CAD build for the part. Positions are in the model's coordinates, mm. A direction names the side the tool comes from. Coordinates: 2 decimals unless noted, no trailing zeros. Write each loop counter-clockwise with the first axis right and the second up, starting at its lowest first coordinate (ties: lowest second). Pieces come first, ordered by that corner, then holes. Notation, with made-up numbers: (-34.75, 42.25) - (-20.75, 42.25) arc R27 cw to (-20.75, 76.25) - close; hole circle Ø2 at (47, 70). An arc over 180 degrees is marked (long way). Answer in a Markdown table with one row per item. Add a question column.
Q1. Band-saw the part on C-C (z = -10.75). List the corners of the cut face in (x, y) (3 decimals), and give its area (3 significant figures).
Q2. Two-plate mould, pull along X, no slides. Class faces 1 (the flat face through (-3, 27.813, -10)), 2 (the cylindrical face through (-4.48, 29.42, -2.52)), 3 (the flat face through (0, 34, -10)): +X half, -X half, draft (parallel to the pull), parting line (faces both ways), or undercut.
Q3. 3-axis set-ups, long thin cutter, end or side, ignore diameter. For faces 4 (the flat face through (0, 14, -10)), 5 (the flat face through (-3, 30.988, -10)), 6 (the flat face through (40.005, 14, -10)): which of +Z, -Z, +X, -X, +Y, -Y reach the whole face in a straight line?
Q4. Band-saw the part on A-A (z = -5.25). List the corners of the cut face in (x, y) (3 decimals).
Q5. Pin check, flat tips, straight feed: pin 1 (10 mm diameter, centred on y = 6, z = -6, fed in from +X) (3 decimals); pin 2 (5 mm diameter, centred on x = 24.5, y = 21, fed in from +Z); pin 3 (5 mm diameter, centred on x = 28, z = -12, fed in from +Y); pin 4 (4 mm diameter, centred on y = 24.5, z = -15, fed in from -X). Stop position of each tip, or through.
Q6. Band-saw the part on D-D (x = 11). List the corners of the cut face in (y, z), and give its area (3 significant figures).
Q7. Drill centre lines: line 1 along Y through (x, z) = (25, -4.25); line 2 along X through (y, z) = (16, -18.5) (3 decimals); line 3 along Y through (x, z) = (43, -18.5). Where is each one in solid material? Low to high. Write a range as from..to.
Q8. Band-saw the part on B-B (y = 19). List the corners of the cut face in (x, z) (3 decimals).
```python
from build123d import *

# Parameters (mm, degrees)
SKETCH1_W           = 40.005
SKETCH1_H           = 19.939
BOSS_EXTRUDE1_DEPTH = 37.338
SKETCH2_W           = 19.939
SKETCH2_H           = 3.175
BOSS_EXTRUDE2_DEPTH = 7.62
SKETCH3_R           = 2.2225
CUT_EXTRUDE1_DEPTH  = 61.215948801
SKETCH4_R           = 2.921
BOSS_EXTRUDE3_DEPTH = 8.636


with BuildPart() as part:
    # Sketch1 → Boss-Extrude1 (new body)
    with BuildSketch(Plane(origin=(0, 0, 0), x_dir=(1, 0, 0), z_dir=(0, 1, 0))):
        with Locations((20.0025, 9.9695)):
            Rectangle(SKETCH1_W, SKETCH1_H)
    extrude(amount=BOSS_EXTRUDE1_DEPTH)

    # Sketch2 → Boss-Extrude2 (add)
    with BuildSketch(Plane(origin=(40.005, 0, 0), x_dir=(0, 0, -1), z_dir=(1, 0, 0))):
        with Locations((9.9695, 29.4005)):
            Rectangle(SKETCH2_W, SKETCH2_H)
    boss_extrude2 = extrude(amount=BOSS_EXTRUDE2_DEPTH)

    # Sketch3 → Cut-Extrude1 (cut, through all)
    with BuildSketch(Plane(origin=(0, 30.988, 0), x_dir=(1, 0, 0), z_dir=(0, 1, 0))):
        with Locations(Location((45.339, 15.367, 0), (0, 0, 270))):
            Circle(SKETCH3_R)
        with Locations(Location((45.339, 4.572, 0), (0, 0, 270))):
            Circle(SKETCH3_R)
    cut_extrude1 = extrude(amount=-CUT_EXTRUDE1_DEPTH, mode=Mode.SUBTRACT)

    # Mirror1: Boss-Extrude2, Cut-Extrude1 across plane
    add(boss_extrude2.mirror(Plane(origin=(20.0025, 0, 0), x_dir=(0, 0, 1), z_dir=(1, 0, 0))))
    add(cut_extrude1.mirror(Plane(origin=(20.0025, 0, 0), x_dir=(0, 0, 1), z_dir=(1, 0, 0))), mode=Mode.SUBTRACT)

    # Sketch4 → Boss-Extrude3 (add)
    with BuildSketch(Plane(origin=(0, 37.338, 0), x_dir=(1, 0, 0), z_dir=(0, 1, 0))):
        with Locations(Location((9.779, 9.9695, 0), (0, 0, 90))):
            Circle(SKETCH4_R)
    extrude(amount=BOSS_EXTRUDE3_DEPTH)


solid = part.part
```
Checked values:
| question | item | result |
|---|---|---|
| 1 | outline | (-7.62, 27.813) - (0, 27.813) - (0, 0) - (40.005, 0) - (40.005, 27.813) - (47.625, 27.813) - (47.625, 30.988) - (40.005, 30.988) - (40.005, 37.338) - (12.594, 37.338) - (12.594, 45.974) - (6.964, 45.974) - (6.964, 37.338) - (0, 37.338) - (0, 30.988) - (-7.62, 30.988) - close |
| 1 | area | 1,590 mm² |
| 2 | face 1 | draft |
| 2 | face 2 | undercut |
| 2 | face 3 | -X half |
| 3 | face 4 | +Z, -Z, -X, -Y |
| 3 | face 5 | +Z, -Z, -X, +Y |
| 3 | face 6 | +Z, -Z, +X, -Y |
| 4 | outline | (-7.62, 27.813) - (-7.451, 27.813) - (-7.451, 30.988) - (-7.62, 30.988) - close; (-3.217, 27.813) - (0, 27.813) - (0, 0) - (40.005, 0) - (40.005, 27.813) - (43.222, 27.813) - (43.222, 30.988) - (40.005, 30.988) - (40.005, 37.338) - (0, 37.338) - (0, 30.988) - (-3.217, 30.988) - close; (47.456, 27.813) - (47.625, 27.813) - (47.625, 30.988) - (47.456, 30.988) - close |
| 5 | pin 1 | stops at x = 40.005 |
| 5 | pin 2 | stops at z = 0 |
| 5 | pin 3 | stops at y = 37.34 |
| 5 | pin 4 | stops at x = 0 |
| 6 | outline | (0, -19.94) - (37.34, -19.94) - (37.34, -12.62) - (45.97, -12.62) - (45.97, -7.32) - (37.34, -7.32) - (37.34, 0) - (0, 0) - close |
| 6 | area | 790 mm² |
| 7 | line 1 | y = 0..37.34 |
| 7 | line 2 | x = 0..40.005 |
| 7 | line 3 | y = 27.81..30.99 |
| 8 | outline | (0, -19.939) - (40.005, -19.939) - (40.005, 0) - (0, 0) - close |
